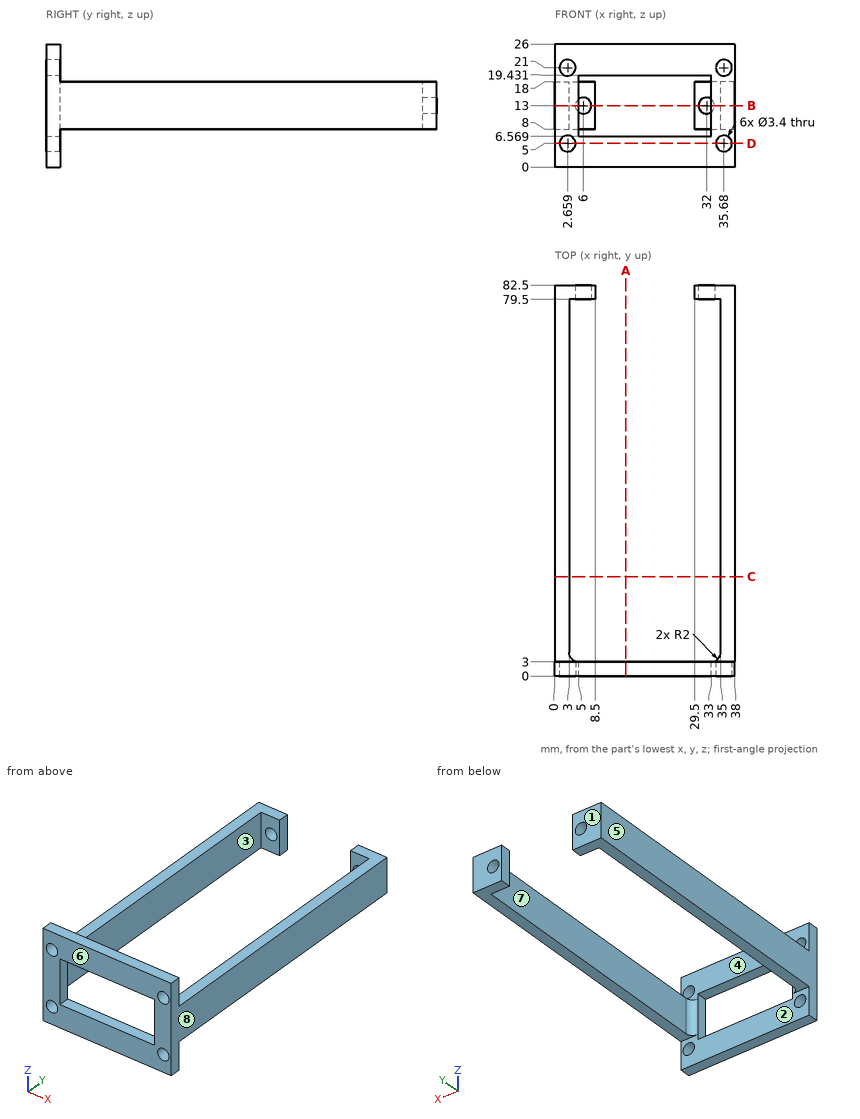
Source: three-view drawing plus pictorial views. Frame: mm from the lowest corner of the part. A direction names the side the tool comes from. Coordinates: 2 decimals unless noted, no trailing zeros. Write each loop counter-clockwise with the first axis right and the second up, starting at its lowest first coordinate (ties: lowest second). Pieces come first, ordered by that corner, then holes. Notation, with made-up numbers: (3.5, -32) - (41.5, -32) arc R9 cw to (41.5, -28) - close; hole circle Ø3 at (21.25, 73.5). An arc over 180 degrees is marked (long way). Return JSON: item names as keys, results as strings.
Item 1: Section query C-C (y = 21). Output: boundary loops of the cut face in (x, z).
Completed:
{"outline": "(0, 8) - (3, 8) - (3, 18) - (0, 18) - close; (35, 8) - (38, 8) - (38, 18) - (35, 18) - close"}
Item 2: Pin query (flat end, axial travel): pin 1 Ø9.5 at (x, y) = (4, 36.5) entering from +Z; pin 2 Ø3 at (x, z) = (30, 14) entering from -Y; pin 3 Ø2.5 at (x, z) = (17.5, 5) entering from +Y. Return the tip coordinate at first contact, or that it passes through.
Completed:
{"pin 1": "stops at z = 18", "pin 2": "stops at y = 79.5", "pin 3": "stops at y = 3"}
Item 3: Section query A-A (x = 15). Output: boundary loops of the cut face in (y, z).
Completed:
{"outline": "(0, 0) - (3, 0) - (3, 6.57) - (0, 6.57) - close; (0, 19.43) - (3, 19.43) - (3, 26) - (0, 26) - close"}
Item 4: Reachability of the marked faces 1, 2, 3, 4 and 5 from +Z, -Z, +X, -X, +Y, -Y: full face, straight path, thin tool, end or side. Return the list, or none.
Completed:
{"face 1": "+Z, -Z, +X, -X, +Y", "face 2": "-Z, +X, -X, +Y", "face 3": "+Z, -Z", "face 4": "+Z, +X, -X, +Y", "face 5": "+Z, -Z, -X, +Y, -Y"}
Item 5: Section query D-D (z = 5). Output: boundary loops of the cut face in (x, y).
Completed:
{"outline": "(0, 0) - (0.96, 0) - (0.96, 3) - (0, 3) - close; (4.36, 0) - (33.98, 0) - (33.98, 3) - (4.36, 3) - close; (37.38, 0) - (38, 0) - (38, 3) - (37.38, 3) - close"}
Item 6: Pull-direction query (Y, two-part tool) for the marked faces 6, 7 and 8; classes: +Y half, -Y half, draft (parallel to the pull), parting line (faces both ways), or undercut.
Completed:
{"face 6": "-Y half", "face 7": "undercut", "face 8": "draft"}
Item 7: Line query: L1, parallel to X at y = 80.6, z = 13; L2, parallel to X at y = 2.3, z = 21; L3, parallel to X at y = 23, z = 14.75. Output: solid intervals per line, ascending.
Completed:
{"L1": "x = 0 to 4.3, 7.7 to 8.5, 29.5 to 30.3, 33.7 to 38", "L2": "x = 0 to 0.96, 4.36 to 33.98, 37.38 to 38", "L3": "x = 0 to 3, 35 to 38"}
Item 8: Section query B-B (z = 13). Output: boundary loops of the cut face in (x, y).
Completed:
{"outline": "(0, 0) - (5, 0) - (5, 3) arc R2 cw to (3, 5) - (3, 79.5) - (4.3, 79.5) - (4.3, 82.5) - (0, 82.5) - close; (7.7, 79.5) - (8.5, 79.5) - (8.5, 82.5) - (7.7, 82.5) - close; (29.5, 79.5) - (30.3, 79.5) - (30.3, 82.5) - (29.5, 82.5) - close; (33, 0) - (38, 0) - (38, 82.5) - (33.7, 82.5) - (33.7, 79.5) - (35, 79.5) - (35, 5) arc R2 cw to (33, 3) - close"}
